The model under review builds one solid part; all positions refer to its coordinate system, in mm. A direction names the side the tool comes from. Coordinates: 2 decimals unless noted, no trailing zeros. Order: outer loops, then holes, each group sorted by start corner. A loop starts at its lowest first (then second) coordinate and runs counter-clockwise, first axis right, second up. Notation, with made-up numbers: M 82.25,-23.5 L 89.25,-23.5 A5 cw 89.25,-15.5 Z; hole C 27,38 d7. An arc over 180 degrees is marked long. Answer as CSV lines item,"result". Start each with the question number.
Q1. Consider section C-C on x = 1123.5. Write out the cut boundary in (y, z).
Q2. Wall thickness on L1, parallel to X at y = 67.5, z = 1175.5; L2, parallel to Z at x = 1384, y = 178.5; L3, parallel to Z at x = 1106.5, y = 99.5: over which ranges is each line inside the solid? List them lowest first. Write a range as [from, to].
Q3. Consider section A-A on z = 1241. Write out the cut boundary in (x, y), and give its area (3 significant figures).
Q4. The part is to be moulded in two halves that separate along Z. For faces 6 (the face through (1301.419, 93.916, 758.113)), 7 (the face through (1291.599, 93.916, 1299.205)), 8 (the face through (530, 152.527, 120)), say which applies: +Z half, -Z half, draft (parallel to the pull), parting line (faces both ways), or undercut.
Q5. For P1, Ø12, axis at x = 691, y = 130, coming from the +Z side; P2, Ø1, axis at x = 284.5, z = 483.5, coming from the +Y side; P3, Ø2, axis at y = 120, z = 949.5, coming from the +X side, all flat-tipped, find the tip position at first contact; note any pin that passes through.
Q6. Consider section D-D on z = 922. Write out the cut boundary in (x, y), and give its area (3 significant figures).
Q7. Machinability: for faces 1 (the face through (957, 152.527, 132)), 2 (the face through (954, 190.5, 1012)), 3 (the face through (239.072, 93.916, 1274.101)), 4 (the face through (773, 0, 773)), 5 (the face through (213.99, 171.18, 1173.46)), which of the approach directions +Z, -Z, +X, -X, +Y, -Y give a long, thin tool a straight path to every point of the face, cutting with its end or side? Answer none if there is none.
Q8. Consider section B-B on y = 45. Write out the cut boundary in (x, z).
from build123d import *

# Parameters (mm, degrees)
BOSS_EXTRUDE1_DEPTH = 152.4
CUT_EXTRUDE1_DEPTH  = 152.4
BOSS_EXTRUDE2_DEPTH = 38.1
BOSS_EXTRUDE3_DEPTH = 190.5
BOSS_EXTRUDE4_DEPTH = 768.35
SKETCH9_R           = 152.4
SKETCH9_R_2         = 146.05
SKETCH9_R_3         = 63.5
SKETCH9_R_4         = 57.15
SKETCH9_W           = 88.9
SKETCH9_H           = 88.9
BOSS_EXTRUDE5_DEPTH = 0.127


with BuildPart() as part:
    # Sketch2 → Boss-Extrude1 (new body)
    with BuildSketch(Plane(origin=(0, 0, 0), x_dir=(1, 0, 0), z_dir=(0, 1, 0))):
        Polygon((0, 0), (0, -1513.1731564), (1513.1731564, 0), align=None)
    extrude(amount=BOSS_EXTRUDE1_DEPTH)

    # Sketch3 → Cut-Extrude1 (cut)
    with BuildSketch(Plane(origin=(0, 152.4, 0), x_dir=(1, 0, 0), z_dir=(0, 1, 0))):
        with BuildLine():
            Line((0, 0), (304.8, 0))
            ThreePointArc((304.8, 0), (215.526146906, -215.526146906), (0, -304.8))
            Line((0, -304.8), (0, 0))
        make_face()
    extrude(amount=-CUT_EXTRUDE1_DEPTH, mode=Mode.SUBTRACT)

    # Sketch4 → Boss-Extrude2 (add)
    with BuildSketch(Plane(origin=(0, 152.4, 0), x_dir=(1, 0, 0), z_dir=(0, 1, 0))):
        Polygon((0, -1513.1731564), (1513.1731564, 0), (1387.449570705, 0), (0, -1387.449570705), align=None)
    extrude(amount=BOSS_EXTRUDE2_DEPTH)

    # Sketch5 → Boss-Extrude3 (add)
    with BuildSketch(Plane(origin=(0, 0, 0), x_dir=(1, 0, 0), z_dir=(0, 1, 0))):
        Polygon((1028.239325862, -484.933830538), (484.933830538, -1028.239325862), (1023.749197802, -1567.054693127), (1567.054693127, -1023.749197802), align=None)
    extrude(amount=BOSS_EXTRUDE3_DEPTH)

    # Sketch6 → Boss-Extrude4 (add)
    with BuildSketch(Plane(origin=(-271.652747662, 0, 271.652747662), x_dir=(0.7071067811865476, 0, 0.7071067811865476), z_dir=(-0.7071067811865476, 0, 0.7071067811865476))):
        Polygon((981.075, 190.5), (841.375, 152.4), (981.075, 152.4), align=None)
    extrude(amount=-BOSS_EXTRUDE4_DEPTH)

    # Sketch9 → Boss-Extrude5 (add)
    # profile 1 of 6: a face of its own
    with BuildSketch(Plane(origin=(0, 152.4, 0), x_dir=(1, 0, 0), z_dir=(0, 1, 0))):
        with Locations(Location((947.417020773, -188.585378542, 0), (0, 0, 270))):
            Circle(SKETCH9_R)
        with Locations(Location((947.417020773, -188.585378542, 0), (0, 0, 270))):
            Circle(SKETCH9_R_2, mode=Mode.SUBTRACT)
    # profile 2 of 6: a face of its own
    with BuildSketch(Plane(origin=(0, 152.4, 0), x_dir=(1, 0, 0), z_dir=(0, 1, 0))):
        with Locations(Location((947.417020773, -188.585378542, 0), (0, 0, 270))):
            Circle(SKETCH9_R_3)
        with Locations(Location((947.417020773, -188.585378542, 0), (0, 0, 270))):
            Circle(SKETCH9_R_4, mode=Mode.SUBTRACT)
    # profile 3 of 6: a face of its own
    with BuildSketch(Plane(origin=(0, 152.4, 0), x_dir=(1, 0, 0), z_dir=(0, 1, 0))):
        with Locations(Location((188.585378542, -947.417020773, 0), (0, 0, 270))):
            Circle(SKETCH9_R)
        with Locations(Location((188.585378542, -947.417020773, 0), (0, 0, 270))):
            Circle(SKETCH9_R_2, mode=Mode.SUBTRACT)
    # profile 4 of 6: a face of its own
    with BuildSketch(Plane(origin=(0, 152.4, 0), x_dir=(1, 0, 0), z_dir=(0, 1, 0))):
        with Locations(Location((188.585378542, -947.417020773, 0), (0, 0, 270))):
            Circle(SKETCH9_R_3)
        with Locations(Location((188.585378542, -947.417020773, 0), (0, 0, 270))):
            Circle(SKETCH9_R_4, mode=Mode.SUBTRACT)
    # profile 5 of 6: a face of its own
    with BuildSketch(Plane(origin=(0, 152.4, 0), x_dir=(1, 0, 0), z_dir=(0, 1, 0))):
        with Locations((530.199570705, -120.65)):
            Rectangle(SKETCH9_W, SKETCH9_H)
    # profile 6 of 6: a face of its own
    with BuildSketch(Plane(origin=(0, 152.4, 0), x_dir=(1, 0, 0), z_dir=(0, 1, 0))):
        with Locations((120.65, -530.199570705)):
            Rectangle(SKETCH9_W, SKETCH9_H)
    extrude(amount=BOSS_EXTRUDE5_DEPTH)


solid = part.part
Evaluation:
1,outline,"M 0,0 L 152.4,0 L 152.4,263.95 L 190.5,263.95 L 190.5,389.67 L 0,389.67 Z; M 0,580.19 L 190.5,580.19 L 190.5,1467.3 L 0,1467.3 Z"
2,L1,"x = [0, 337.67], [632.19, 1415.3]"
2,L2,"z = [3.45, 129.17], [840.69, 1206.8]"
2,L3,"z = [0, 406.67], [563.19, 1484.3]"
3,outline,"M 0,0 L 272.17,0 L 272.17,190.5 L 146.45,190.5 L 146.45,152.4 L 0,152.4 Z; M 697.69,0 L 1349.8,0 L 1349.8,190.5 L 697.69,190.5 Z"
3,area,"170,000 mm²"
4,face 6,"undercut"
4,face 7,"+Z half"
4,face 8,"draft"
5,P1,"stops at z = 1240.31"
5,P2,"stops at y = 152.4"
5,P3,"stops at x = 1493.81"
6,outline,"M 0,0 L 1465.31,0 L 1465.31,190.5 L 465.45,190.5 L 378.69,173.77 L 378.69,152.4 L 338.85,152.4 L 338.85,152.53 L 332.41,152.53 L 332.41,152.4 L 246.78,152.4 L 246.78,152.53 L 239.77,152.53 L 239.77,152.4 L 137.4,152.4 L 137.4,152.53 L 130.39,152.53 L 130.39,152.4 L 44.76,152.4 L 44.76,152.53 L 38.32,152.53 L 38.32,152.4 L 0,152.4 Z"
6,area,"264,000 mm²"
7,face 1,"-Z, -X, +Y"
7,face 2,"+Z, -Z, +X, -X, +Y"
7,face 3,"+Z, +Y, -Y"
7,face 4,"+Z, -Z, +X, -X, -Y"
7,face 5,"-X, +Y"
8,outline,"M 0,304.8 A304.8 cw 304.8,0 L 1513.17,0 L 1028.24,484.93 L 1567.05,1023.75 L 1023.75,1567.05 L 484.93,1028.24 L 0,1513.17 Z"
